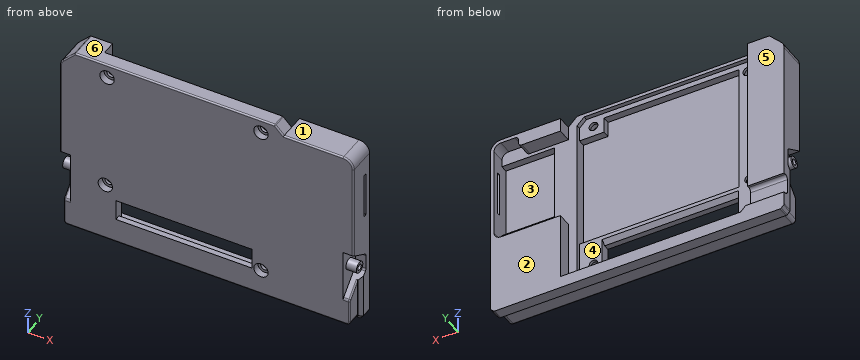
from build123d import *

# Parameters (mm, degrees)
SKETCH_1_W           = 84
SKETCH_1_H           = 54
EXTRUDE_1_DEPTH      = 8
SKETCH_2_W           = 60
SKETCH_2_H           = 2.5
EXTRUDE_2_DEPTH      = 8
CHAMFER_1_SIZE       = 4
FILLET_1_R           = 3
SKETCH_3_W           = 1
SKETCH_3_H           = 4
CUT_EXTRUDE_1_DEPTH  = 101.179838291
CUT_EXTRUDE_2_DEPTH  = 1.1
CUT_EXTRUDE_START    = -84
CUT_EXTRUDE_3_DEPTH  = 1.1
FILLET_2_R           = 1
CHAMFER_2_SIZE       = 1
CUT_EXTRUDE_4_DEPTH  = 1.9
CUT_EXTRUDE_START_2  = -81.8
CUT_EXTRUDE_5_DEPTH  = 1.9
FILLET_3_R           = 1
CHAMFER_4_SIZE       = 1
SKETCH_6_R           = 1.6
EXTRUDE_3_DEPTH      = 3
EXTRUDE_START        = -81
SKETCH_6_2_R         = 1.6
EXTRUDE_4_DEPTH      = 3
SKETCH_7_R           = 0.85
CUT_EXTRUDE_6_DEPTH  = 7
CUT_EXTRUDE_START_3  = -77
SKETCH_7_2_R         = 0.85
CUT_EXTRUDE_7_DEPTH  = 7
FILLET_4_R           = 0.5
SKETCH_8_W           = 53.5
SKETCH_8_H           = 53
CUT_EXTRUDE_8_DEPTH  = 4
CUT_EXTRUDE_9_DEPTH  = 1.2
CHAMFER_5_SIZE       = 2
SKETCH_11_R          = 1.25
CUT_EXTRUDE_10_DEPTH = 100.995199885
CUT_EXTRUDE_13_DEPTH = 101.179838291
FILLET_5_R           = 0.4
FILLET_6_R           = 0.4
CUT_EXTRUDE_14_DEPTH = 2
SKETCH_16_W          = 39
SKETCH_16_H          = 6
CUT_EXTRUDE_15_DEPTH = 101.179838291
CHAMFER_6_SIZE       = 1.2
SKETCH_17_W          = 14
SKETCH_17_H          = 6
CUT_EXTRUDE_16_DEPTH = 1.6
CUT_EXTRUDE_18_DEPTH = 4
SKETCH_21_W          = 15
SKETCH_21_H          = 22
CUT_EXTRUDE_19_DEPTH = 2
OTHER_1_OUTLINE_R    = 2.05
OTHER_1_OUTLINE_R_2  = 1.25
OTHER_1_DEPTH        = 2
FILLET_8_R           = 1
CUT_EXTRUDE_20_REACH = 102.18


# Read off the part's stored shape, not the designer's step: 高级异型孔1
# Some blends are built 0.0001 mm under size
with BuildPart() as part:
    # 草图1 → 凸台-拉伸1 (new body)
    with BuildSketch(Plane(origin=(0, 0, 0), x_dir=(1, 0, 0), z_dir=(0, 1, 0))):
        with Locations((42, 27)):
            Rectangle(SKETCH_1_W, SKETCH_1_H)
    extrude(amount=EXTRUDE_1_DEPTH)

    # 草图2 → 凸台-拉伸2 (add)
    with BuildSketch(Plane.XZ):
        with Locations((30, 1.25)):
            Rectangle(SKETCH_2_W, SKETCH_2_H)
    extrude(amount=-EXTRUDE_2_DEPTH)

    # 倒角1
    # the kernel refuses this chamfer: 4 mm, written as the material it adds along each edge
    with BuildSketch(Plane(origin=(60, 0, 0), x_dir=(0.9996219169112968, 0, -0.02749587661058639), z_dir=(0, 1, 0))) as chamfer_1_piece_1_section:
        Polygon((CHAMFER_1_SIZE * 0.999621916911, -CHAMFER_1_SIZE * 0.0274958766106), (-CHAMFER_1_SIZE * 0.0274958766106, -CHAMFER_1_SIZE * 0.999621916911), (0, 0), align=None)
    chamfer_1_piece_1 = extrude(amount=8, mode=Mode.PRIVATE)
    chamfer_1_piece_1 = split(chamfer_1_piece_1, bisect_by=Plane(origin=(61.48305822, 4, 2.5), z_dir=(0, 0, -1)), keep=Keep.TOP, mode=Mode.PRIVATE)
    add(chamfer_1_piece_1)

    # 圆角1
    fillet_1_edges = [part.edges().sort_by_distance(p)[0] for p in [
        (84, 4, 0),
    ]]
    fillet(fillet_1_edges, radius=FILLET_1_R)

    # 草图3 → 切除-拉伸1 (cut, through all)
    with BuildSketch(Plane.ZY):
        with Locations((-53.5, 2)):
            Rectangle(SKETCH_3_W, SKETCH_3_H)
    extrude(amount=-CUT_EXTRUDE_1_DEPTH, mode=Mode.SUBTRACT)

    # 草图4 → 切除-拉伸2 (cut)
    with BuildSketch(Plane.ZY):
        Polygon((-34, 6.2), (-30.420428331, 0), (-53, 0), (-53, 4), (-41.2, 4), (-39, 6.2), align=None)
    extrude(amount=-CUT_EXTRUDE_2_DEPTH, mode=Mode.SUBTRACT)

    # 草图4<3> → 切除-拉伸3 (cut)
    with BuildSketch(Plane.ZY.offset(CUT_EXTRUDE_START)):
        Polygon((-34, 6.2), (-30.420428331, 0), (-53, 0), (-53, 4), (-41.2, 4), (-39, 6.2), align=None)
    extrude(amount=CUT_EXTRUDE_3_DEPTH, mode=Mode.SUBTRACT)

    # 圆角2
    fillet_2_edges = [part.edges().sort_by_distance(p)[0] for p in [
        (1.1, 2, -53),
        (82.9, 2, -53),
    ]]
    fillet(fillet_2_edges, radius=FILLET_2_R)

    # 倒角2
    chamfer_2_edges = [part.edges().sort_by_distance(p)[0] for p in [
        (0, 6, -54),
        (84, 6, -54),
    ]]
    chamfer(chamfer_2_edges, length=CHAMFER_2_SIZE)

    # 草图5 → 切除-拉伸4 (cut)
    with BuildSketch(Plane.ZY.offset(-1.1)):
        Polygon((-45.2, 0), (-30.420428331, 0), (-34, 6.2), (-39, 6.2), align=None)
    extrude(amount=-CUT_EXTRUDE_4_DEPTH, mode=Mode.SUBTRACT)

    # 草图5<2> → 切除-拉伸5 (cut)
    with BuildSketch(Plane.ZY.offset(-1.1).offset(CUT_EXTRUDE_START_2)):
        Polygon((-39, 6.2), (-41.2, 4), (-45.2, 0), (-30.420428331, 0), (-34, 6.2), align=None)
    extrude(amount=CUT_EXTRUDE_5_DEPTH, mode=Mode.SUBTRACT)

    # 圆角3
    fillet_3_edges = [part.edges().sort_by_distance(p)[0] for p in [
        (2.05, 0, -45.2),
        (81.95, 0, -45.2),
        (1.5, 6.2, -39),
        (1.5, 6.2, -34),
        (82.5, 6.2, -34),
        (82.5, 6.2, -39),
    ]]
    fillet(fillet_3_edges, radius=FILLET_3_R)

    # 倒角4
    chamfer_4_edges = [part.edges().sort_by_distance(p)[0] for p in [
        (42, 4, -54),
        (83.5, 4, -53.5),
        (0.5, 4, -53.5),
        (84, 4, -47.1),
        (0, 4, -47.1),
    ]]
    chamfer(chamfer_4_edges, length=CHAMFER_4_SIZE - 0.0001)  # a hair under: the kernel refuses the full size

    # 草图6 → 凸台-拉伸3 (add)
    with BuildSketch(Plane.ZY.offset(-3)):
        with Locations((-36, 3)):
            Circle(SKETCH_6_R)
    extrude(amount=EXTRUDE_3_DEPTH)

    # 草图6<2> → 凸台-拉伸4 (add)
    with BuildSketch(Plane.ZY.offset(-3).offset(EXTRUDE_START)):
        with Locations((-36, 3)):
            Circle(SKETCH_6_2_R)
    extrude(amount=EXTRUDE_4_DEPTH)

    # 草图7 → 切除-拉伸6 (cut)
    with BuildSketch(Plane.ZY):
        with Locations((-36, 3)):
            Circle(SKETCH_7_R)
    extrude(amount=-CUT_EXTRUDE_6_DEPTH, mode=Mode.SUBTRACT)

    # 草图7<2> → 切除-拉伸7 (cut)
    with BuildSketch(Plane.ZY.offset(CUT_EXTRUDE_START_3)):
        with Locations((-36, 3)):
            Circle(SKETCH_7_2_R)
    extrude(amount=-CUT_EXTRUDE_7_DEPTH, mode=Mode.SUBTRACT)

    # 圆角4
    fillet_4_edges = [part.edges().sort_by_distance(p)[0] for p in [
        (0, 6.49995, -53),
        (83, 6.49995, -54),
        (1, 6.49995, -54),
        (84, 6.49995, -53),
    ]]
    fillet(fillet_4_edges, radius=FILLET_4_R)

    # 草图8 → 切除-拉伸8 (cut)
    with BuildSketch(Plane(origin=(0, 8, 0), x_dir=(1, 0, 0), z_dir=(0, 1, 0))):
        with Locations((37.25, 24)):
            Rectangle(SKETCH_8_W, SKETCH_8_H)
    extrude(amount=-CUT_EXTRUDE_8_DEPTH, mode=Mode.SUBTRACT)

    # 草图10 → 切除-拉伸9 (cut)
    with BuildSketch(Plane(origin=(0, 4, 0), x_dir=(1, 0, 0), z_dir=(0, 1, 0))):
        Polygon((10.5, -1.5), (59.5, -1.5), (61.5, 0.5), (61.5, 50.5), (10.5, 50.5), align=None)
    extrude(amount=-CUT_EXTRUDE_9_DEPTH, mode=Mode.SUBTRACT)

    # 倒角5
    chamfer_5_edges = [part.edges().sort_by_distance(p)[0] for p in [
        (10.5, 5.4, -50.5),
    ]]
    chamfer(chamfer_5_edges, length=CHAMFER_5_SIZE)

    # 草图11 → 切除-拉伸10 (cut, through all)
    with BuildSketch(Plane(origin=(0, 2.8, 0), x_dir=(1, 0, 0), z_dir=(0, 1, 0))):
        with Locations(Location((13.5, 1.5, 0), (0, 0, 270))):
            Circle(SKETCH_11_R)
        with Locations(Location((57.5, 1.5, 0), (0, 0, 270))):
            Circle(SKETCH_11_R)
        with Locations(Location((57.5, 45.5, 0), (0, 0, 270))):
            Circle(SKETCH_11_R)
        with Locations(Location((13, 36, 0), (0, 0, 270))):
            Circle(SKETCH_11_R)
    extrude(amount=-CUT_EXTRUDE_10_DEPTH, mode=Mode.SUBTRACT)

    # 草图14 → 切除-拉伸13 (cut, through all)
    with BuildSketch(Plane(origin=(0, 8, 0), x_dir=(1, 0, 0), z_dir=(0, 1, 0))):
        with BuildLine():
            Line((4.257359313, -2.5), (0, -2.5))
            Line((0, -2.5), (0, 3))
            ThreePointArc((0, 3), (0.228361402, 1.851949703), (0.878679656, 0.878679656))
            Line((0.878679656, 0.878679656), (4.257359313, -2.5))
        make_face()
    extrude(amount=-CUT_EXTRUDE_13_DEPTH, mode=Mode.SUBTRACT)

    # 圆角5
    fillet_5_edges = [part.edges().sort_by_distance(p)[0] for p in [
        (61.5, 2, 2.5),
        (4.257359313, 4, 2.5),
    ]]
    fillet(fillet_5_edges, radius=FILLET_5_R)

    # 圆角6
    fillet_6_edges = [part.edges().sort_by_distance(p)[0] for p in [
        (82.9, 2.146446609, -43.053553391),
        (82.9, 0.076120467, -45.23153013),
        (1.1, 2.146446609, -43.053553391),
        (1.1, 0.076120467, -45.23153013),
        (72.5, 0, 0),
        (62.808578644, 0, 1.191421356),
        (0.228361402, 0, -1.851949703),
        (32.878679656, 0, 2.5),
        (84, 0, -16.710214166),
        (2.509440841, 0, 0.752081528),
        (4.269971365, 0, 2.469551813),
        (61.487387948, 0, 2.469551813),
        (83.121320344, 0, -0.878679656),
        (0, 0, -16.710214166),
        (1.1, 0, -48.807106781),
        (82.9, 0, -48.807106781),
        (42, 0, -53),
        (82.607106781, 0, -52.707106781),
        (1.392893219, 0, -52.707106781),
    ]]
    fillet(fillet_6_edges, radius=FILLET_6_R)

    # 草图15 → 切除-拉伸14 (cut)
    with BuildSketch(Plane(origin=(0, 2.8, 0), x_dir=(1, 0, 0), z_dir=(0, 1, 0))):
        Polygon((15.9, 37.5), (61.5, 37.5), (61.5, 4.5), (54.5, 4.5), (54.5, 0), (15.9, 0), align=None)
    extrude(amount=-CUT_EXTRUDE_14_DEPTH, mode=Mode.SUBTRACT)

    # 草图16 → 切除-拉伸15 (cut, through all)
    with BuildSketch(Plane.XZ):
        with Locations((35.5, -42.8)):
            Rectangle(SKETCH_16_W, SKETCH_16_H)
    extrude(amount=-CUT_EXTRUDE_15_DEPTH, mode=Mode.SUBTRACT)

    # 倒角6
    chamfer_6_edges = [part.edges().sort_by_distance(p)[0] for p in [
        (35.5, 2.8, -39.8),
        (35.5, 2.8, -45.8),
    ]]
    chamfer(chamfer_6_edges, length=CHAMFER_6_SIZE)

    # 草图17 → 切除-拉伸16 (cut)
    with BuildSketch(Plane(origin=(0, 8, 0), x_dir=(1, 0, 0), z_dir=(0, 1, 0))):
        with Locations((7, 46)):
            Rectangle(SKETCH_17_W, SKETCH_17_H)
    extrude(amount=-CUT_EXTRUDE_16_DEPTH, mode=Mode.SUBTRACT)

    # 草图20 → 切除-拉伸18 (cut)
    with BuildSketch(Plane(origin=(0, 8, 0), x_dir=(1, 0, 0), z_dir=(0, 1, 0))):
        with BuildLine():
            Line((64, 31), (81, 31))
            ThreePointArc((81, 31), (82.414213562, 30.414213562), (83, 29))
            Line((83, 29), (83, 3))
            ThreePointArc((83, 3), (82.414213562, 1.585786438), (81, 1))
            Line((81, 1), (77, 1))
            ThreePointArc((77, 1), (76.292893219, 1.292893219), (76, 2))
            Line((76, 2), (76, 3))
            ThreePointArc((76, 3), (75.707106781, 3.707106781), (75, 4))
            Line((75, 4), (64, 4))
            Line((64, 4), (64, 31))
        make_face()
    extrude(amount=-CUT_EXTRUDE_18_DEPTH, mode=Mode.SUBTRACT)

    # 草图21 → 切除-拉伸19 (cut)
    with BuildSketch(Plane(origin=(0, 4, 0), x_dir=(1, 0, 0), z_dir=(0, 1, 0))):
        with Locations((75.5, 16)):
            Rectangle(SKETCH_21_W, SKETCH_21_H)
    extrude(amount=-CUT_EXTRUDE_19_DEPTH, mode=Mode.SUBTRACT)

    # 高级异型孔1 outline → 高级异型孔1 (cut)
    # profile 1 of 4: a face of its own
    with BuildSketch(Plane(origin=(0, 0, 0), x_dir=(1, 0, 0), z_dir=(0, 1, 0))):
        with Locations((13, 36)):
            Circle(OTHER_1_OUTLINE_R)
        with Locations((13, 36)):
            Circle(OTHER_1_OUTLINE_R_2, mode=Mode.SUBTRACT)
    # profile 2 of 4: a face of its own
    with BuildSketch(Plane(origin=(0, 0, 0), x_dir=(1, 0, 0), z_dir=(0, 1, 0))):
        with Locations((13.5, 1.5)):
            Circle(OTHER_1_OUTLINE_R)
        with Locations((13.5, 1.5)):
            Circle(OTHER_1_OUTLINE_R_2, mode=Mode.SUBTRACT)
    # profile 3 of 4: a face of its own
    with BuildSketch(Plane(origin=(0, 0, 0), x_dir=(1, 0, 0), z_dir=(0, 1, 0))):
        with Locations((57.5, 1.5)):
            Circle(OTHER_1_OUTLINE_R)
        with Locations((57.5, 1.5)):
            Circle(OTHER_1_OUTLINE_R_2, mode=Mode.SUBTRACT)
    # profile 4 of 4: a face of its own
    with BuildSketch(Plane(origin=(0, 0, 0), x_dir=(1, 0, 0), z_dir=(0, 1, 0))):
        with Locations((57.5, 45.5)):
            Circle(OTHER_1_OUTLINE_R)
        with Locations((57.5, 45.5)):
            Circle(OTHER_1_OUTLINE_R_2, mode=Mode.SUBTRACT)
    extrude(amount=OTHER_1_DEPTH, mode=Mode.SUBTRACT)

    # 圆角8
    fillet_8_edges = [part.edges().sort_by_distance(p)[0] for p in [
        (5.25, 6.4, -43),
        (5.5, 6.4, -49),
    ]]
    fillet(fillet_8_edges, radius=FILLET_8_R)

    # 草图24 → 切除-拉伸20 (cut, up to next)
    with BuildSketch(Plane(origin=(84, 0, 0), x_dir=(0, 0, -1), z_dir=(1, 0, 0)), mode=Mode.PRIVATE) as cut_extrude_20_sk1:
        Polygon((21.4, 5.3), (15.4, 5.3), (14.4, 5.3), (8.4, 5.3), (8.4, 6.3), (14.4, 6.3), (15.4, 6.3), (21.4, 6.3), align=None)
    cut_extrude_20_tool1 = extrude(cut_extrude_20_sk1.sketch, amount=-CUT_EXTRUDE_20_REACH, mode=Mode.PRIVATE) & part.part
    add(cut_extrude_20_tool1.solids().sort_by_distance((84, 5.8, -14.9))[0], mode=Mode.SUBTRACT)


solid = part.part
Part model, mm, in its own coordinate system. Face numbers are marked on the shaded views. A direction names the side the tool comes from. Give positions to 0.01 mm unless a question says otherwise; leave off trailing zeros. Order: outer loops, then holes, each group sorted by start corner. A loop starts at its lowest first (then second) coordinate and runs counter-clockwise, first axis right, second up. Notation, with made-up numbers: (81, -24) - (94, -24) arc R18 ccw to (94, -6) - close; hole circle Ø2 at (-1.75, -4). An arc over 180 degrees is marked (long way). One line per question, with ' | ' between items.
1. Drill centre lines: probe 1 along X at (y, z) = (2.35, -45.5); probe 2 along Z at (x, y) = (57.5, 0.4); probe 3 along Z at (x, y) = (57.5, 2.5). Where is each one in solid material? Low to high.
Filled in:
probe 1: 1.1 to 16, 55 to 56.25, 58.75 to 82.9 | probe 2: -53 to -47.55, -43.45 to -3.55, 0.55 to 2.5 | probe 3: -53 to -46.75, -44.25 to -37.5, -4.5 to -2.75, -0.25 to 2.5
2. Which spindle directions (+Z, -Z, +X, -X, +Y, -Y) get a long thin tool onto all of the face, cutting with end or side? Do the marked faces 1, 2 and 3. Say none if no direction does.
Filled in:
face 1: +Z, +X, +Y, -Y | face 2: +Z, -Z, +X, -X, +Y | face 3: +Y
3. Band-saw the part on C-C on z = -6. List the corners of the cut face in (x, y), then the cut area to 3 significant figures.
Filled in:
outline: (0, 0.4) arc R0.4 ccw to (0.4, 0) - (83.6, 0) arc R0.4 ccw to (84, 0.4) - (84, 8) - (83, 8) - (83, 2) - (68, 2) - (68, 4) - (61.5, 4) - (61.5, 0.8) - (15.9, 0.8) - (15.9, 2.8) - (10.5, 2.8) - (10.5, 8) - (0, 8) - close | area: 200 mm²
4. Band-saw the part on B-B on z = -12. List the corners of the cut face in (x, y).
Filled in:
outline: (0, 0.4) arc R0.4 ccw to (0.4, 0) - (83.6, 0) arc R0.4 ccw to (84, 0.4) - (84, 5.3) - (83, 5.3) - (83, 2) - (68, 2) - (68, 4) - (61.5, 4) - (61.5, 0.8) - (15.9, 0.8) - (15.9, 2.8) - (10.5, 2.8) - (10.5, 8) - (0, 8) - close; (83, 6.3) - (84, 6.3) - (84, 8) - (83, 8) - close
5. Drop flat-ended pins along their axis: P1, Ø10, axis at x = 48.5, z = -30.5, coming from the +Y side; P2, Ø3.5, axis at x = 13, z = -36, coming from the -Y side; P3, Ø1.1, axis at x = 83.5, y = 5.5, coming from the +Z side. Give the stop position or say it passes through.
Filled in:
P1: y = 0.8 | P2: y = 2 | P3: z = -0.72
6. Pull direction Z, two halves, no side cores. Call the marked faces 4, 5 and 6: +Z half, -Z half, draft (parallel to the pull), parting line (faces both ways), or undercut.
Filled in:
face 4: undercut | face 5: draft | face 6: +Z half
